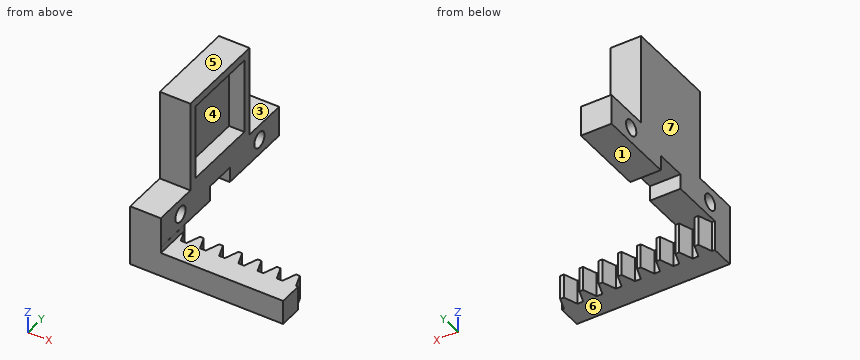
```python
from build123d import *

# Parameters (mm, degrees)
BLANKSKE_W          = 31.75
BLANKSKE_H          = 7.62
BLANK_DEPTH         = 6.35
TOOTHCUTSIM_DEPTH   = 34.263334168
TEETHCUTS_COUNT     = 9
TEETHCUTS_PITCH     = 3.989822666
SKETCH1_W           = 6.35
SKETCH1_H           = 12.7
BOSS_EXTRUDE1_DEPTH = 6.35
SKETCH2_R           = 1.65
CUT_EXTRUDE1_DEPTH  = 6.35
SKETCH4_W           = 6.35
SKETCH4_H           = 19.05
BOSS_EXTRUDE3_DEPTH = 19.05
SKETCH6_W           = 6.35
SKETCH6_H           = 12.7
BOSS_EXTRUDE5_DEPTH = 6.35
SKETCH7_R           = 1.65
CUT_EXTRUDE2_DEPTH  = 6.35
SKETCH8_W           = 15.748
SKETCH8_H           = 15.748
CUT_EXTRUDE3_DEPTH  = 3.175
SKETCH11_W          = 6.35
SKETCH11_H          = 6.35
BOSS_EXTRUDE7_DEPTH = 12.7
SKETCH12_W          = 3.175
SKETCH12_H          = 6.35
CUT_EXTRUDE4_DEPTH  = 6.35
SKETCH13_W          = 25.382452533
SKETCH13_H          = 7.62
CUT_EXTRUDE5_DEPTH  = 1.27


with BuildPart() as part:
    # BlankSke → Blank (new body)
    with BuildSketch(Plane.XY):
        with Locations((15.875, 3.81)):
            Rectangle(BLANKSKE_W, BLANKSKE_H)
    extrude(amount=-BLANK_DEPTH)

    # TooCutSkeSim → ToothCutSim (cut, through all)
    with BuildSketch(Plane.XY):
        Polygon((0.595165029, 4.826), (-0.595165029, 4.826), (-1.621342708, 7.6454), (1.621342708, 7.6454), align=None)
    toothcutsim = extrude(amount=-TOOTHCUTSIM_DEPTH, mode=Mode.SUBTRACT)

    # TeethCuts: ToothCutSim ×9
    with Locations(*[(i * TEETHCUTS_PITCH, 0, 0) for i in range(1, TEETHCUTS_COUNT)]):
        add(toothcutsim, mode=Mode.SUBTRACT)

    # Sketch1 → Boss-Extrude1 (add)
    with BuildSketch(Plane.XY):
        with Locations((3.175, 6.35)):
            Rectangle(SKETCH1_W, SKETCH1_H)
    extrude(amount=BOSS_EXTRUDE1_DEPTH)

    # Sketch2 → Cut-Extrude1 (cut)
    with BuildSketch(Plane.ZY):
        with Locations((3.175, 6.35)):
            Circle(SKETCH2_R)
    extrude(amount=-CUT_EXTRUDE1_DEPTH, mode=Mode.SUBTRACT)

    # Sketch4 → Boss-Extrude3 (add)
    with BuildSketch(Plane.XY.offset(6.35)):
        with Locations((3.175, 19.05)):
            Rectangle(SKETCH4_W, SKETCH4_H)
    extrude(amount=BOSS_EXTRUDE3_DEPTH)

    # Sketch6 → Boss-Extrude5 (add)
    with BuildSketch(Plane(origin=(6.35, 0, 0), x_dir=(0, 0, -1), z_dir=(1, 0, 0))):
        with Locations((-3.175, 31.75)):
            Rectangle(SKETCH6_W, SKETCH6_H)
    extrude(amount=-BOSS_EXTRUDE5_DEPTH)

    # Sketch7 → Cut-Extrude2 (cut)
    with BuildSketch(Plane(origin=(6.35, 0, 0), x_dir=(0, 0, -1), z_dir=(1, 0, 0))):
        with Locations(Location((-3.175, 31.75, 0), (0, 0, 90))):
            Circle(SKETCH7_R)
    extrude(amount=-CUT_EXTRUDE2_DEPTH, mode=Mode.SUBTRACT)

    # Sketch8 → Cut-Extrude3 (cut)
    with BuildSketch(Plane(origin=(6.35, 0, 0), x_dir=(0, 0, -1), z_dir=(1, 0, 0))):
        with Locations((-15.875, 19.05)):
            Rectangle(SKETCH8_W, SKETCH8_H)
    extrude(amount=-CUT_EXTRUDE3_DEPTH, mode=Mode.SUBTRACT)

    # Sketch11 → Boss-Extrude7 (add)
    with BuildSketch(Plane(origin=(0, 12.7, 0), x_dir=(1, 0, 0), z_dir=(0, 1, 0))):
        with Locations((3.175, -3.175)):
            Rectangle(SKETCH11_W, SKETCH11_H)
    extrude(amount=BOSS_EXTRUDE7_DEPTH)

    # Sketch12 → Cut-Extrude4 (cut)
    with BuildSketch(Plane(origin=(6.35, 0, 0), x_dir=(0, 0, -1), z_dir=(1, 0, 0))):
        with Locations((-1.5875, 19.05)):
            Rectangle(SKETCH12_W, SKETCH12_H)
    extrude(amount=-CUT_EXTRUDE4_DEPTH, mode=Mode.SUBTRACT)

    # Sketch13 → Cut-Extrude5 (cut)
    with BuildSketch(Plane.XY):
        with Locations((19.058773734, 3.81)):
            Rectangle(SKETCH13_W, SKETCH13_H)
    extrude(amount=-CUT_EXTRUDE5_DEPTH, mode=Mode.SUBTRACT)


solid = part.part
```
Geometry check sheet. Reference: the model listing, model coordinates, mm. Face numbers are marked on the shaded views. A direction names the side the tool comes from. Give positions to 0.01 mm unless a question says otherwise; leave off trailing zeros. Order: outer loops, then holes, each group sorted by start corner. A loop starts at its lowest first (then second) coordinate and runs counter-clockwise, first axis right, second up.
1. Thickness scan on L1, parallel to Y at x = 4.5, z = 13 (3 decimals); L2, parallel to Z at x = 4.25, y = 31.75 (3 decimals); L3, parallel to Z at x = 4, y = 31. Record the ranges inside material, lowest first.
2. Section check D-D, the plane x = 24. Enter the section's corners in (y, z), and give its area (3 significant figures).
3. Access from +Z, -Z, +X, -X, +Y, -Y to the whole of each face (thin tool, end or side, straight path). Record for the marked faces 1, 2 and 3.
4. Section check C-C, the plane y = 21.5. Enter the section's corners in (x, z) (3 decimals), and give its area (3 significant figures).
5. Gauge pin test, flat ends, axial feed: pin 1 Ø8 at (y, z) = (21.5, 4) entering from +X; pin 2 Ø8 at (y, z) = (9.5, 2.5) entering from +X; pin 3 Ø2.5 at (x, z) = (5, 19.5) entering from +Y (3 decimals); pin 4 Ø2 at (y, z) = (31.75, 3.175) entering from -X. Record the tip position at first contact, or that the pin passes through.
6. Section check A-A, the plane y = 31.75. Enter the section's corners in (x, z) (3 decimals).
7. Section check B-B, the plane z = 11. Enter the section's corners in (x, y) (3 decimals).
8. Release check for a two-part mould opening along Z. For the marked faces 4, 5, 6 and 7 record: pulls with the +Z half, pulls with the -Z half, needs draft (parallel to the pull), parting line crosses it, or undercut.
Values follow:
1. L1: y = 9.525 to 11.176, 26.924 to 28.575
1. L2: z = 0 to 1.525, 4.825 to 6.35
1. L3: z = 0 to 1.71, 4.64 to 6.35
2. outline: (0, -6.35) - (4.83, -6.35) - (4.83, -1.27) - (0, -1.27) - close
2. area: 24.5 mm2
3. face 1: -Z, +X, -X, +Y
3. face 2: +Z, +X, +Y, -Y
3. face 3: +Z, +X, -X, +Y
4. outline: (0, 3.175) - (6.35, 3.175) - (6.35, 8.001) - (3.175, 8.001) - (3.175, 23.749) - (6.35, 23.749) - (6.35, 25.4) - (0, 25.4) - close
4. area: 91.1 mm2
5. pin 1: stops at x = 6.35
5. pin 2: stops at x = 6.37
5. pin 3: stops at y = 28.575
5. pin 4: passes through
6. outline: (0, 0) - (6.35, 0) - (6.35, 1.525) - (0, 1.525) - close; (0, 4.825) - (6.35, 4.825) - (6.35, 6.35) - (0, 6.35) - close
7. outline: (0, 9.525) - (6.35, 9.525) - (6.35, 11.176) - (3.175, 11.176) - (3.175, 26.924) - (6.35, 26.924) - (6.35, 28.575) - (0, 28.575) - close
8. face 4: undercut
8. face 5: pulls with the +Z half
8. face 6: pulls with the -Z half
8. face 7: needs draft
